from build123d import *

# Parameters (mm, degrees)
SKETCH1_W               = 50.8
SKETCH1_H               = 25.4
SKETCH1_W_2             = 47.625
SKETCH1_H_2             = 22.225
BOSS_EXTRUDE1_DEPTH     = 395.478
CUT_EXTRUDE1_DEPTH      = 400.535540952
CUT_EXTRUDE1_DEPTH_BACK = 400.535540952
SKETCH2_R               = 14.224
SKETCH2_R_2             = 3.175


with BuildPart() as part:
    # Sketch1 → Boss-Extrude1 (new body)
    with BuildSketch(Plane.XY):
        with Locations((25.4, 12.7)):
            Rectangle(SKETCH1_W, SKETCH1_H)
        with Locations((25.4, 12.7)):
            Rectangle(SKETCH1_W_2, SKETCH1_H_2, mode=Mode.SUBTRACT)
    extrude(amount=BOSS_EXTRUDE1_DEPTH)

    # Sketch2 → Cut-Extrude1 (cut, two sides: drawn at the far end of the back side and taken through both)
    with BuildSketch(Plane(origin=(0, 25.4, 0), x_dir=(1, 0, 0), z_dir=(0, 1, 0)).offset(-CUT_EXTRUDE1_DEPTH_BACK)):
        with Locations(Location((25.4, -38.1, 0), (0, 0, 90))):
            Circle(SKETCH2_R)
        with Locations(Location((12.7, -16.102954744, 0), (0, 0, 90))):
            Circle(SKETCH2_R_2)
        with Locations(Location((12.7, -60.097045256, 0), (0, 0, 90))):
            Circle(SKETCH2_R_2)
        with Locations(Location((38.1, -60.097045256, 0), (0, 0, 90))):
            Circle(SKETCH2_R_2)
        with Locations(Location((38.1, -16.102954744, 0), (0, 0, 90))):
            Circle(SKETCH2_R_2)
        with Locations(Location((25.4, -357.378, 0), (0, 0, 90))):
            Circle(SKETCH2_R)
    extrude(amount=CUT_EXTRUDE1_DEPTH + CUT_EXTRUDE1_DEPTH_BACK, mode=Mode.SUBTRACT)


solid = part.part
The model under review builds one solid part; all positions refer to its coordinate system, in mm. A direction names the side the tool comes from. Round coordinates to 2 decimals unless told otherwise and drop trailing zeros. Loops run counter-clockwise (first coordinate to the right, second up) from the corner with the lowest first, then second, coordinate; pieces in that order, holes last. Notation, with made-up numbers: (29.5, 60.5) -> (65.5, 60.5) arc R9 cw to (65.5, 67.5) -> close; hole circle Ø10 at (54.5, 53). An arc over 180 degrees is marked (long way). One line per question, with ' | ' between items. Start each with the question number.
Item 1: Add section C-C, the plane x = 31.5. Write out the cut boundary in (y, z), then the cut area to 3 significant figures.
Item 2: Wall thickness on line 1 along X through (y, z) = (1.2, 38.1); line 2 along X through (y, z) = (2.5, 344.5); line 3 along Y through (x, z) = (21, 207.5): over which ranges is each line inside the solid? List them lowest first. Write a range as [from, to].
Item 3: Add section A-A, the plane z = 38.1. Write out the cut boundary in (x, y).
Item 4: Add section D-D, the plane z = 199. Write out the cut boundary in (x, y).
Item 5: Draft analysis for pull direction X (two halves, no side actions). For faces 1 (the face through (23, 1, 395.478)), 2 (the face through (0, 13, 195)), 3 (the face through (25, 23.812, 195)), state which applies: +X half, -X half, draft (parallel to the pull), parting line (faces both ways), or undercut.
Item 6: Machinability: for faces 4 (the face through (49.212, 13, 195)), 5 (the face through (30.85, 0.78, 344.24)), which of the approach directions +Z, -Z, +X, -X, +Y, -Y give a long, thin tool a straight path to every point of the face, cutting with its end or side? Answer none if there is none.
Item 7: Add section B-B, the plane y = 7. Write out the cut boundary in (x, z).
Return value:
1) outline: (0, 0) -> (1.59, 0) -> (1.59, 25.25) -> (0, 25.25) -> close; (0, 50.95) -> (1.59, 50.95) -> (1.59, 344.53) -> (0, 344.53) -> close; (0, 370.23) -> (1.59, 370.23) -> (1.59, 395.48) -> (0, 395.48) -> close; (23.81, 0) -> (25.4, 0) -> (25.4, 25.25) -> (23.81, 25.25) -> close; (23.81, 50.95) -> (25.4, 50.95) -> (25.4, 344.53) -> (23.81, 344.53) -> close; (23.81, 370.23) -> (25.4, 370.23) -> (25.4, 395.48) -> (23.81, 395.48) -> close | area: 1,090 mm2
2) line 1: x = [0, 11.18], [39.62, 50.8] | line 2: x = [0, 1.59], [49.21, 50.8] | line 3: y = [0, 1.59], [23.81, 25.4]
3) outline: (0, 0) -> (11.18, 0) -> (11.18, 1.59) -> (1.59, 1.59) -> (1.59, 23.81) -> (11.18, 23.81) -> (11.18, 25.4) -> (0, 25.4) -> close; (39.62, 0) -> (50.8, 0) -> (50.8, 25.4) -> (39.62, 25.4) -> (39.62, 23.81) -> (49.21, 23.81) -> (49.21, 1.59) -> (39.62, 1.59) -> close
4) outline: (0, 0) -> (50.8, 0) -> (50.8, 25.4) -> (0, 25.4) -> close; hole (1.59, 1.59) -> (49.21, 1.59) -> (49.21, 23.81) -> (1.59, 23.81) -> close
5) face 1: draft | face 2: -X half | face 3: undercut
6) face 4: +Z, -Z | face 5: +Y, -Y
7) outline: (0, 0) -> (1.59, 0) -> (1.59, 395.48) -> (0, 395.48) -> close; (49.21, 0) -> (50.8, 0) -> (50.8, 395.48) -> (49.21, 395.48) -> close
